Could you check a few things on this model? Use its own coordinates, in mm. Round coordinates to 2 decimals unless told otherwise and drop trailing zeros. Order: outer loops, then holes, each group sorted by start corner. A loop starts at its lowest first (then second) coordinate and runs counter-clockwise, first axis right, second up.
```python
from build123d import *

# Parameters (mm, degrees)
SKETCH1_W           = 88.9
SKETCH1_H           = 25.4
BOSS_EXTRUDE1_DEPTH = 6.35
SKETCH2_R           = 1.016
CUT_EXTRUDE1_DEPTH  = 7.35
SKETCH3_R           = 1.524
CUT_EXTRUDE2_DEPTH  = 7.35


with BuildPart() as part:
    # Sketch1 → Boss-Extrude1 (new body)
    with BuildSketch(Plane.XY):
        with Locations((44.45, 12.7)):
            Rectangle(SKETCH1_W, SKETCH1_H)
    extrude(amount=BOSS_EXTRUDE1_DEPTH)

    # Sketch2 → Cut-Extrude1 (cut, through all)
    with BuildSketch(Plane.XY.offset(6.35)):
        with Locations((7.62, 6.35)):
            Circle(SKETCH2_R)
        with Locations((33.02, 6.35)):
            Circle(SKETCH2_R)
        with Locations((55.88, 6.35)):
            Circle(SKETCH2_R)
        with Locations((81.28, 6.35)):
            Circle(SKETCH2_R)
    extrude(amount=-CUT_EXTRUDE1_DEPTH, mode=Mode.SUBTRACT)

    # Sketch3 → Cut-Extrude2 (cut, through all)
    with BuildSketch(Plane.XY.offset(6.35)):
        with Locations((22.225, 19.05)):
            Circle(SKETCH3_R)
        with Locations((66.675, 19.05)):
            Circle(SKETCH3_R)
    extrude(amount=-CUT_EXTRUDE2_DEPTH, mode=Mode.SUBTRACT)


solid = part.part
```
Q1. Imagine slicing it at A-A, the plane y = 19.05. Please give me the cut outline in (x, z), then the cut area to 3 significant figures.
Q2. We'd pull the mould along Y, two halves only. Please class faces 1 (the flat face through (44, 0, 3)), 2 (the cylindrical face through (82.22, 5.96, 3.22)), 3 (the cylindrical face through (33.96, 5.96, 3.22)), 4 (the flat face through (0, 13, 3)): released by +Y, released by -Y, zero draft, split by the parting line, or undercut.
Q3. Imagine slicing it at B-B, the plane y = 6.35. Please give me the cut outline in (x, z).
Q4. For P1, Ø1.6, axis at x = 55.88, y = 6.35, coming from the +Z side; P2, Ø10, axis at x = 72, y = 5.5, coming from the -Z side, each with a flat end and sliding along its axis, tell me the tip position at first contact or that it passes through.
Q5. Imagine slicing it at C-C, the plane x = 55.88. Please give me the cut outline in (y, z).
Q6. I need wall thicknesses on L1, parallel to X at y = 6.75, z = 6.25; L2, parallel to Y at x = 33.02, z = 4.75; L3, parallel to X at y = 19.5, z = 3.75. Which ranges of each line are inside material? Lowest first, please.
Filled in:
1. outline: (0, 0) - (20.7, 0) - (20.7, 6.35) - (0, 6.35) - close; (23.75, 0) - (65.15, 0) - (65.15, 6.35) - (23.75, 6.35) - close; (68.2, 0) - (88.9, 0) - (88.9, 6.35) - (68.2, 6.35) - close
1. area: 526 mm2
2. face 1: released by -Y
2. face 2: undercut
2. face 3: undercut
2. face 4: zero draft
3. outline: (0, 0) - (6.6, 0) - (6.6, 6.35) - (0, 6.35) - close; (8.64, 0) - (32, 0) - (32, 6.35) - (8.64, 6.35) - close; (34.04, 0) - (54.86, 0) - (54.86, 6.35) - (34.04, 6.35) - close; (56.9, 0) - (80.26, 0) - (80.26, 6.35) - (56.9, 6.35) - close; (82.3, 0) - (88.9, 0) - (88.9, 6.35) - (82.3, 6.35) - close
4. P1: passes through
4. P2: stops at z = 0
5. outline: (0, 0) - (5.33, 0) - (5.33, 6.35) - (0, 6.35) - close; (7.37, 0) - (25.4, 0) - (25.4, 6.35) - (7.37, 6.35) - close
6. L1: x = 0 to 6.69, 8.55 to 32.09, 33.95 to 54.95, 56.81 to 80.35, 82.21 to 88.9
6. L2: y = 0 to 5.33, 7.37 to 25.4
6. L3: x = 0 to 20.77, 23.68 to 65.22, 68.13 to 88.9
